from build123d import *

# Parameters (mm, degrees)
ESBO_O1_W                  = 320
ESBO_O1_H                  = 170
RESSALTO_EXTRUS_O1_DEPTH   = 12
ESBO_O2_R                  = 4.5
CORTE_EXTRUS_O1_DEPTH      = 1
CORTE_EXTRUS_O1_DEPTH_BACK = 13


with BuildPart() as part:
    # Esboço1 → Ressalto-extrusão1 (new body)
    with BuildSketch(Plane(origin=(0, 0, 0), x_dir=(1, 0, 0), z_dir=(0, 1, 0))):
        Rectangle(ESBO_O1_W, ESBO_O1_H)
    extrude(amount=RESSALTO_EXTRUS_O1_DEPTH)

    # Esboço2 → Corte-extrusão1 (cut, two sides)
    with BuildSketch(Plane(origin=(0, 12, 0), x_dir=(1, 0, 0), z_dir=(0, 1, 0))) as corte_extrus_o1_sk:
        with Locations((-23.05, 0)):
            Circle(ESBO_O2_R)
        with Locations((23.05, 0)):
            Circle(ESBO_O2_R)
    extrude(amount=CORTE_EXTRUS_O1_DEPTH, mode=Mode.SUBTRACT)
    extrude(corte_extrus_o1_sk.sketch, amount=-CORTE_EXTRUS_O1_DEPTH_BACK, mode=Mode.SUBTRACT)


solid = part.part
For this review, take the finished solid that the model builds, in its own axes (mm). Round coordinates to 2 decimals unless told otherwise and drop trailing zeros. Write each loop counter-clockwise with the first axis right and the second up, starting at its lowest first coordinate (ties: lowest second). Pieces come first, ordered by that corner, then holes. Notation, with made-up numbers: (-37.75, 62.25) - (17.25, 62.25) arc R33 cw to (17.25, 98.25) - close; hole circle Ø1 at (17.5, 68.25). An arc over 180 degrees is marked (long way). Write item = value, one per line. Start each with the question number.
1. Draft analysis for pull direction Z (two halves, no side actions). For faces 1 (the face through (-2, 6, 85)), 2 (the face through (-2, 0, -1)), 3 (the face through (18.554, 6.084, -0.198)), state which applies: released by +Z, released by -Z, zero draft, split by the parting line, or undercut.
2. Wall thickness on L1, parallel to X at y = 8.25, z = 0; L2, parallel to Z at x = -23.05, y = 6.25; L3, parallel to X at y = 3.75, z = -1: over which ranges is each line inside the solid? List them lowest first.
3. Consider section B-B on x = 23.05. State the section outline as (y, z) points, plus the area to 3 significant figures.
4. For pin 1 Ø1.5 at (x, z) = (-10.5, -38.5) entering from -Y; pin 2 Ø8 at (x, z) = (-23.05, 0) entering from -Y, all flat-tipped, find the tip position at first contact; note any pin that passes through.
5. Consider section A-A on z = 0. State the section outline as (x, y) points, plus the area to 3 significant figures.
Evaluation:
q1.face_1 = released by +Z
q1.face_2 = zero draft
q1.face_3 = undercut
q2.L1 = -160 to -27.55, -18.55 to 18.55, 27.55 to 160
q2.L2 = -85 to -4.5, 4.5 to 85
q2.L3 = -160 to -27.44, -18.66 to 18.66, 27.44 to 160
q3.outline = (0, -85) - (12, -85) - (12, -4.5) - (0, -4.5) - close; (0, 4.5) - (12, 4.5) - (12, 85) - (0, 85) - close
q3.area = 1,930 mm2
q4.pin_1 = 0
q4.pin_2 = through
q5.outline = (-160, 0) - (-27.55, 0) - (-27.55, 12) - (-160, 12) - close; (-18.55, 0) - (18.55, 0) - (18.55, 12) - (-18.55, 12) - close; (27.55, 0) - (160, 0) - (160, 12) - (27.55, 12) - close
q5.area = 3,620 mm2
